Work out the finished part from the listing and answer in its coordinate system (mm). A direction names the side the tool comes from. Give positions to 0.01 mm unless a question says otherwise; leave off trailing zeros. Write each loop counter-clockwise with the first axis right and the second up, starting at its lowest first coordinate (ties: lowest second). Pieces come first, ordered by that corner, then holes. Notation, with made-up numbers: (50.25, -4) - (87.25, -4) arc R15 cw to (87.25, 12) - close; hole circle Ø7 at (6.5, 32.25). An arc over 180 degrees is marked (long way). Write item = value, one per line.
from build123d import *

# Parameters (mm, degrees)
SKETCH1_W           = 40.7
SKETCH1_H           = 36.2
BOSS_EXTRUDE1_DEPTH = 20
SKETCH2_W           = 6.55
SKETCH2_H           = 2.2
BOSS_EXTRUDE2_DEPTH = 20
SKETCH3_R           = 6.25
BOSS_EXTRUDE3_DEPTH = 38.8
SKETCH3_3_R         = 6.25
SKETCH3_3_R_2       = 2.75
SKETCH3_3_R_3       = 1.6
BOSS_EXTRUDE4_DEPTH = 40.1
SKETCH3_4_R         = 2.75
SKETCH3_4_R_2       = 1.6
BOSS_EXTRUDE5_DEPTH = 42.7
SKETCH5_R           = 2.5
CUT_EXTRUDE1_DEPTH  = 43.9
SKETCH8_R           = 2.5
CUT_EXTRUDE2_DEPTH  = 43.9
SKETCH10_R          = 2.5
CUT_EXTRUDE3_DEPTH  = 43.9
SKETCH12_W          = 7
SKETCH12_H          = 1.5
BOSS_EXTRUDE6_DEPTH = 6


with BuildPart() as part:
    # Sketch1 → Boss-Extrude1 (new body)
    with BuildSketch(Plane(origin=(0, 0, 0), x_dir=(0, 0, -1), z_dir=(1, 0, 0))):
        with Locations((-15.995997066, 21.093377017)):
            Rectangle(SKETCH1_W, SKETCH1_H)
    extrude(amount=BOSS_EXTRUDE1_DEPTH)

    # Sketch2 → Boss-Extrude2 (add)
    with BuildSketch(Plane(origin=(0, 0, 0), x_dir=(0, 0, -1), z_dir=(1, 0, 0))):
        with Locations((-39.620997066, 30.893377017)):
            Rectangle(SKETCH2_W, SKETCH2_H)
        with Locations((7.629002934, 30.893377017)):
            Rectangle(SKETCH2_W, SKETCH2_H)
    extrude(amount=BOSS_EXTRUDE2_DEPTH)

    # Sketch3 → Boss-Extrude3 (add)
    with BuildSketch(Plane(origin=(0, 2.993377017, 0), x_dir=(1, 0, 0), z_dir=(0, 1, 0))):
        with BuildLine():
            Line((1.4, -10.748937395), (1.4, -32.945997066))
            Line((1.4, -32.945997066), (18.6, -32.945997066))
            Line((18.6, -32.945997066), (18.6, -10.748937395))
            ThreePointArc((18.6, -10.748937395), (10, 4.354002934), (1.4, -10.748937395))
        make_face()
        with Locations(Location((10, -5.645997066, 0), (0, 0, 90))):
            Circle(SKETCH3_R, mode=Mode.SUBTRACT)
    extrude(amount=BOSS_EXTRUDE3_DEPTH)

    # Sketch3<3> → Boss-Extrude4 (add)
    # profile 1 of 2: a face of its own
    with BuildSketch(Plane(origin=(0, 2.993377017, 0), x_dir=(1, 0, 0), z_dir=(0, 1, 0))):
        with Locations(Location((10, -5.645997066, 0), (0, 0, 90))):
            Circle(SKETCH3_3_R)
        with Locations(Location((10, -5.645997066, 0), (0, 0, 90))):
            Circle(SKETCH3_3_R_2, mode=Mode.SUBTRACT)
    # profile 2 of 2: a face of its own
    with BuildSketch(Plane(origin=(0, 2.993377017, 0), x_dir=(1, 0, 0), z_dir=(0, 1, 0))):
        with Locations(Location((10, -5.645997066, 0), (0, 0, 90))):
            Circle(SKETCH3_3_R_3)
    extrude(amount=BOSS_EXTRUDE4_DEPTH)

    # Sketch3<4> → Boss-Extrude5 (add)
    with BuildSketch(Plane(origin=(0, 2.993377017, 0), x_dir=(1, 0, 0), z_dir=(0, 1, 0))):
        with Locations(Location((10, -5.645997066, 0), (0, 0, 90))):
            Circle(SKETCH3_4_R)
        with Locations(Location((10, -5.645997066, 0), (0, 0, 90))):
            Circle(SKETCH3_4_R_2, mode=Mode.SUBTRACT)
    extrude(amount=BOSS_EXTRUDE5_DEPTH)

    # Sketch5 → Cut-Extrude1 (cut)
    with BuildSketch(Plane(origin=(0, 0, 0), x_dir=(1, 0, 0), z_dir=(0, 1, 0))):
        with Locations((15, -40.895997066)):
            Circle(SKETCH5_R)
    extrude(amount=CUT_EXTRUDE1_DEPTH, mode=Mode.SUBTRACT)

    # Sketch8 → Cut-Extrude2 (cut)
    with BuildSketch(Plane(origin=(0, 31.993377017, 0), x_dir=(1, 0, 0), z_dir=(0, 1, 0))):
        with Locations((5, -40.895997066)):
            Circle(SKETCH8_R)
    extrude(amount=-CUT_EXTRUDE2_DEPTH, mode=Mode.SUBTRACT)

    # Sketch10 → Cut-Extrude3 (cut)
    with BuildSketch(Plane(origin=(0, 0, 0), x_dir=(1, 0, 0), z_dir=(0, 1, 0))):
        with Locations((5, 8.904002934)):
            Circle(SKETCH10_R)
        with Locations((15, 8.904002934)):
            Circle(SKETCH10_R)
    extrude(amount=CUT_EXTRUDE3_DEPTH, mode=Mode.SUBTRACT)

    # Sketch12 → Boss-Extrude6 (add)
    with BuildSketch(Plane.XY.offset(36.345997066)):
        with Locations((10, 9.743377017)):
            Rectangle(SKETCH12_W, SKETCH12_H)
        with Locations((10, 8.243377017)):
            Rectangle(SKETCH12_W, SKETCH12_H)
    extrude(amount=BOSS_EXTRUDE6_DEPTH)


solid = part.part
1. For a pull along X with two mould halves and no side action, classify faces 1 (the flat face through (10, 43.093, 6)), 2 (the flat face through (10, 31, -10.904)), 3 (the cylindrical face through (16.1, 42.4, 7)) as pulls with the +X half, pulls with the -X half, needs draft (parallel to the pull), parting line crosses it, or undercut.
Solution:
face_1 = undercut
face_2 = needs draft
face_3 = parting line crosses it
2. Find section C-C, the plane y = 6.5. Give the vertices of the cut face in (x, z), then the cut area to 3 significant figures.
Solution:
outline = (0, -4.35) - (20, -4.35) - (20, 36.35) - (0, 36.35) - close
area = 814 mm^2
3. A tool of negligible diameter and unlimited length cuts with its end or side. For faces 4 (the flat face through (10, 10.493, 39)), 5 (the flat face through (18.6, 40, 22)), 6 (the flat face through (10, 36, 36.346)), 7 (the cylindrical face through (7.68, 44.38, 4.17)), from which of +Z, -Z, +X, -X, +Y, -Y can it reach the whole face along a straight path? Write none if from no direction.
Solution:
face_4 = +Z, +X, -X
face_5 = +Z, +X, +Y
face_6 = +Z, +X, -X, +Y
face_7 = +Y
4. Given pin 1 (12 mm diameter, centred on x = 4, y = 37.5, fed in from +Z); pin 2 (7 mm diameter, centred on x = 9.5, z = 39, fed in from +Y); pin 3 (10 mm diameter, centred on x = 7, y = 15, fed in from +Z); pin 4 (7 mm diameter, centred on x = 12.5, z = -8, fed in from +Y), each flat-ended and moving along its own axis, determine where each tip first touches the part or whether it passes through.
Solution:
pin_1 = 42.9
pin_2 = 39.19
pin_3 = 42.35
pin_4 = 31.99
5. Straight lines are drawn through the part: line 1 (Z direction, x = 10, y = 44.1); line 2 (Y direction, x = 10.75, z = 20.5); line 3 (Z direction, x = 5.25, y = 7.5). For each, find the intervals that lie inside material, in ascending order.
Solution:
line_1 = 2.9 to 4.05, 7.25 to 8.4
line_2 = 2.99 to 41.79
line_3 = -4.35 to 36.35
6. Find section A-A, the plane z = 2. Give the vertices of the cut face in (x, y), then the cut area to 3 significant figures.
Solution:
outline = (0, 2.99) - (20, 2.99) - (20, 39.19) - (19.31, 39.19) - (19.31, 41.79) - (15.08, 41.79) - (15.08, 43.09) - (4.92, 43.09) - (4.92, 41.79) - (0.69, 41.79) - (0.69, 39.19) - (0, 39.19) - close
area = 786 mm^2
7. Find section B-B, the plane x = 5. Give the vertices of the cut face in (y, z), then the cut area to 3 significant figures.
Solution:
outline = (2.99, -4.35) - (29.79, -4.35) - (29.79, -6.4) - (31.99, -6.4) - (31.99, -4.35) - (39.19, -4.35) - (39.19, -3.01) - (41.79, -3.01) - (41.79, 1.9) - (43.09, 1.9) - (43.09, 9.4) - (41.79, 9.4) - (41.79, 32.95) - (39.19, 32.95) - (39.19, 36.35) - (31.99, 36.35) - (31.99, 38.4) - (29.79, 38.4) - (29.79, 36.35) - (2.99, 36.35) - close
area = 1,590 mm^2
